Geometry check sheet. Reference: the model listing, model coordinates, mm. Face numbers are marked on the shaded views. A direction names the side the tool comes from. Round coordinates to 2 decimals unless told otherwise and drop trailing zeros. Write each loop counter-clockwise with the first axis right and the second up, starting at its lowest first coordinate (ties: lowest second). Pieces come first, ordered by that corner, then holes. Notation, with made-up numbers: (22, 62.5) - (60, 62.5) arc R18 ccw to (60, 92.5) - close; hole circle Ø3 at (-7.5, 54.25). An arc over 180 degrees is marked (long way). Return JSON: item names as keys, results as strings. Group by question number.
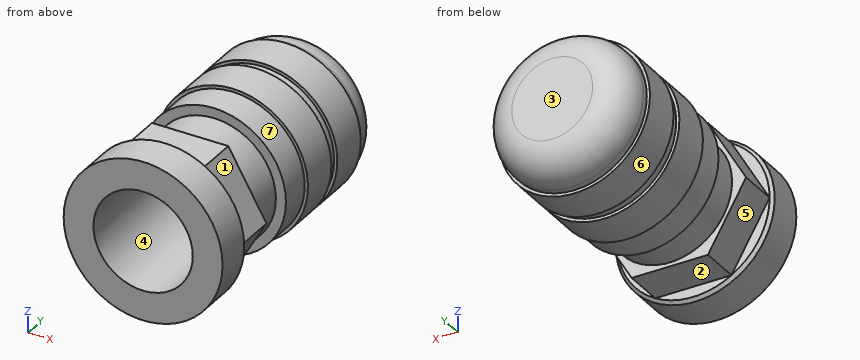
from build123d import *

# Parameters (mm, degrees)
SKETCH1_R      = 6.35
EXTRUDE1_DEPTH = 3.175
CHAMFER1_SIZE  = 0.254
EXTRUDE2_DEPTH = 3.175
SKETCH5_R      = 3.96875
EXTRUDE4_DEPTH = 12.7


with BuildPart() as part:
    # Sketch1 → Extrude1 (new body)
    with BuildSketch(Plane(origin=(0, 0, 0), x_dir=(1, 0, 0), z_dir=(0, 1, 0))):
        Circle(SKETCH1_R)
    extrude(amount=-EXTRUDE1_DEPTH)

    # Chamfer1
    chamfer1_edges = [part.edges().sort_by_distance(p)[0] for p in [
        (-6.35, 0, 0),
    ]]
    chamfer(chamfer1_edges, length=CHAMFER1_SIZE)

    # Sketch2 → Extrude2 (add)
    with BuildSketch(Plane(origin=(0, 0, 0), x_dir=(-1, 0, 0), z_dir=(0, 1, 0))):
        Polygon((-6.096, 0), (-3.048, -5.279290861), (3.048, -5.279290861), (6.096, 0), (3.048, 5.279290861), (-3.048, 5.279290861), align=None)
    extrude(amount=EXTRUDE2_DEPTH)

    # Sketch4 → Revolve1 (revolve)
    with BuildSketch(Plane(origin=(0, 0, 0), x_dir=(0, 0, -1), z_dir=(1, 0, 0))):
        with BuildLine():
            Line((-4.97229944, 3.175), (-4.97229944, 6.35))
            Line((-4.97229944, 6.35), (-5.772606153, 6.35))
            Line((-5.772606153, 6.35), (-5.772606153, 8.887450179))
            Line((-5.772606153, 8.887450179), (-6.026606153, 8.887450179))
            Line((-6.026606153, 8.887450179), (-6.026606153, 12.062450179))
            Line((-6.026606153, 12.062450179), (-5.772606153, 12.062450179))
            Line((-5.772606153, 12.062450179), (-5.772606153, 12.856200179))
            Line((-5.772606153, 12.856200179), (-6.026606153, 12.856200179))
            Line((-6.026606153, 12.856200179), (-6.026606153, 16.031200179))
            Line((-6.026606153, 16.031200179), (-5.772606153, 16.031200179))
            Line((-5.772606153, 16.031200179), (-5.772606153, 16.51))
            ThreePointArc((-5.772606153, 16.51), (-5.028657378, 18.306051224), (-3.232606153, 19.05))
            Line((-3.232606153, 19.05), (0, 19.05))
            Line((0, 19.05), (0, 17.78))
            Line((0, 17.78), (-3.232606153, 17.78))
            ThreePointArc((-3.232606153, 17.78), (-4.130631766, 17.408025612), (-4.502606153, 16.51))
            Line((-4.502606153, 16.51), (-4.502606153, 14.761200179))
            Line((-4.502606153, 14.761200179), (-4.756606153, 14.761200179))
            Line((-4.756606153, 14.761200179), (-4.756606153, 14.126200179))
            Line((-4.756606153, 14.126200179), (-4.502606153, 14.126200179))
            Line((-4.502606153, 14.126200179), (-4.502606153, 10.792450179))
            Line((-4.502606153, 10.792450179), (-4.756606153, 10.792450179))
            Line((-4.756606153, 10.792450179), (-4.756606153, 10.157450179))
            Line((-4.756606153, 10.157450179), (-4.502606153, 10.157450179))
            Line((-4.502606153, 10.157450179), (-4.502606153, 7.62))
            Line((-4.502606153, 7.62), (-3.70229944, 7.62))
            Line((-3.70229944, 7.62), (-3.70229944, 4.445))
            Line((-3.70229944, 4.445), (0, 4.445))
            Line((0, 4.445), (0, 3.175))
            Line((0, 3.175), (-4.97229944, 3.175))
        make_face()
    revolve(axis=Axis((0, 20.169611013, 0), (0, -1, 0)))

    # Sketch5 → Extrude4 (cut)
    with BuildSketch(Plane.XZ.offset(3.175)):
        Circle(SKETCH5_R)
    extrude(amount=-EXTRUDE4_DEPTH, mode=Mode.SUBTRACT)


solid = part.part
1. Section check A-A (y = -2). Enter the section's corners in (x, z), and give its area (3 significant figures).
2. Depth check by flat-ended pin: pin 1 Ø1.9 at (x, z) = (1, -1) entering from -Y; pin 2 Ø3.5 at (x, y) = (-1.5, 2) entering from +Z; pin 3 Ø0.9 at (x, z) = (-5, 2) entering from +Y. Enter the tip coordinate at first touch or a pass-through.
3. Material ranges on line 1 along X through (y, z) = (11.6, 0); line 2 along Z through (x, y) = (0, 3.75); line 3 along Z through (x, y) = (0, 16.1), recorded low to high.
4. Mould release check, pull along Z, two halves, no side actions. Record for the marked faces 1, 2, 3 and 4: pulls with the +Z half, pulls with the -Z half, needs draft (parallel to the pull), parting line crosses it, or undercut.
5. Tool access check on the marked faces 5, 6 and 7. Record the directions out of +Z, -Z, +X, -X, +Y, -Y that give a thin tool (end or side, any length) a straight path to the whole face; none if there is none.
6. Section check B-B (y = 17). Enter the section's corners in (x, z), and give its area (3 significant figures).
Result sheet:
{
 "1": {"outline": "circle Ø12.7 at (0, 0); hole circle Ø7.94 at (0, 0)", "area": "77.2 mm²"},
 "2": {"pin 1": "stops at y = 17.78", "pin 2": "stops at z = 5.28", "pin 3": "stops at y = 18.39"},
 "3": {"line 1": "x = -6.03 to -4.5, 4.5 to 6.03", "line 2": "z = -4.97 to -3.97, 3.97 to 4.97", "line 3": "z = -5.77 to -4.5, 4.5 to 5.77"},
 "4": {"face 1": "pulls with the +Z half", "face 2": "pulls with the -Z half", "face 3": "needs draft", "face 4": "undercut"},
 "5": {"face 5": "-Z, -X", "face 6": "+Y", "face 7": "none"},
 "6": {"outline": "circle Ø11.45 at (0, 0); hole circle Ø8.81 at (0, 0)", "area": "42.0 mm²"}
}
